Check sheet for the modelled part. Datum: model origin and axes. Units: mm. Coordinates: 2 decimals unless noted, no trailing zeros. Loops run counter-clockwise (first coordinate to the right, second up) from the corner with the lowest first, then second, coordinate; pieces in that order, holes last. Notation, with made-up numbers: (13, -16) -> (23, -16) arc R22 cw to (23, 6) -> close; hole circle Ø2 at (1, 72). An arc over 180 degrees is marked (long way). Use CSV: the item, a comma, the result in double quotes. Start each with the question number.
1. Sectioned sample at D-D, the plane z = 3.25. Record the cut outline in (x, y).
2. Sectioned sample at B-B, the plane z = 15. Record the cut outline in (x, y).
3. Sectioned sample at A-A, the plane x = 65. Record the cut outline in (y, z).
4. Sectioned sample at C-C, the plane y = 18. Record the cut outline in (x, z).
5. Thickness scan on L1, parallel to Z at x = 65, y = 36; L2, parallel to X at y = 13.5, z = 11; L3, parallel to Y at x = 20.5, z = 24.5. Record the ranges inside material, lowest first.
6. Release check for a two-part mould opening along Z. For faces 1 (the face through (0, 11, 15)), 2 (the face through (69, 25, 12)), 3 (the face through (49, 20, 30)) record: pulls with the +Z half, pulls with the -Z half, needs draft (parallel to the pull), parting line crosses it, or undercut.
7. Gauge pin test, flat ends, axial feed: pin 1 (4 mm diameter, centred on x = 82.5, z = 3, fed in from +Y); pin 2 (6 mm diameter, centred on x = 37.5, z = 16.5, fed in from +Y); pin 3 (1.5 mm diameter, centred on x = 14.5, z = 16, fed in from +Y). Record the tip position at first contact, or that the pin passes through.
```python
from build123d import *

# Parameters (mm, degrees)
PAD_DEPTH    = 30
SKETCH001_R  = 5
POCKET_DEPTH = 50


with BuildPart() as part:
    # Sketch → Pad (new body)
    with BuildSketch(Plane.XY):
        with BuildLine():
            Line((0, 0), (100, 0))
            Line((100, 0), (100, 30))
            ThreePointArc((100, 30), (94.142136, 44.142136), (80, 50))
            Line((50, 50), (80, 50))
            Line((0, 21.132487), (50, 50))
            Line((0, 21.132487), (0, 0))
        make_face()
    extrude(amount=PAD_DEPTH)

    # Sketch001 (on Face4 of Pad) → Pocket (cut)
    with BuildSketch(Plane(origin=(0, 50, 0), x_dir=(-1, 0, 0), z_dir=(0, 1, 0))):
        with Locations((-65, 15)):
            Circle(SKETCH001_R)
    extrude(amount=-POCKET_DEPTH, mode=Mode.SUBTRACT)


solid = part.part
```
Completed:
1,outline,"(0, 0) -> (100, 0) -> (100, 30) arc R20 ccw to (80, 50) -> (50, 50) -> (0, 21.13) -> close"
2,outline,"(0, 0) -> (60, 0) -> (60, 50) -> (50, 50) -> (0, 21.13) -> close; (70, 0) -> (100, 0) -> (100, 30) arc R20 ccw to (80, 50) -> (70, 50) -> close"
3,outline,"(0, 0) -> (50, 0) -> (50, 10) -> (0, 10) -> close; (0, 20) -> (50, 20) -> (50, 30) -> (0, 30) -> close"
4,outline,"(0, 0) -> (100, 0) -> (100, 30) -> (0, 30) -> close; hole circle Ø10 at (65, 15)"
5,L1,"0 to 10, 20 to 30"
5,L2,"0 to 62, 68 to 100"
5,L3,"0 to 32.97"
6,face 1,"needs draft"
6,face 2,"undercut"
6,face 3,"pulls with the +Z half"
7,pin 1,"y = 49.99"
7,pin 2,"y = 44.52"
7,pin 3,"y = 29.94"
